Work out the finished part from the listing and answer in its coordinate system (mm). A direction names the side the tool comes from. Round coordinates to 2 decimals unless told otherwise and drop trailing zeros.
1. Flat-ended cylindrical pins translate along their axes: pin 1 Ø0.5 at (x, z) = (0, -3) entering from +Y; pin 2 Ø1.8 at (x, z) = (-2, -2) entering from +Y; pin 3 Ø4 at (x, y) = (2.5, 11.5) entering from -Z. Find the tip coordinate at first contact, or state that the pin passes through.
2. Straight lines are drawn through the part: probe 1 along X at (y, z) = (12, 2); probe 2 along X at (y, z) = (57.5, -2.25); probe 3 along Z at (x, y) = (-0.5, 27.5). For each, find the intervals that lie inside material, in ascending order.
3. A tool of negligible diameter and unlimited length cuts with its end or side. For faces 1 (the face through (-3, 0, 2)), 2 (the face through (-3, 60, 2)), 3 (the face through (3, 0, 2)), 4 (the face through (3, 60, -2)), from which of +Z, -Z, +X, -X, +Y, -Y can it reach the whole face along a straight path? Write none if from no direction.
```python
from build123d import *
from build123d.topology import SkipClean

# Parameters (mm, degrees)
BOSS_EXTRUDE1_DEPTH = 60
SKETCH4_R           = 2.375
BOSS_EXTRUDE3_DEPTH = 2
FILLET1_R           = 0.5
BOSS_EXTRUDE5_START = 2
SKETCH6_R           = 2.375
BOSS_EXTRUDE5_DEPTH = 2
FILLET2_R           = 1


with BuildPart() as part:
    # Sketch2 → Boss-Extrude1 (new body)
    with BuildSketch(Plane(origin=(0, 0, 0), x_dir=(1, 0, 0), z_dir=(0, 1, 0))):
        with BuildLine():
            Line((3.775215965, -0.978645895), (2.300774305, -0.58912019))
            ThreePointArc((2.300774305, -0.58912019), (2.374963211, 0.013219106), (2.294073837, 0.614695232))
            Line((2.294073837, 0.614695232), (3.742962577, 1.0029238))
            ThreePointArc((3.742962577, 1.0029238), (3.356294138, 1.936727823), (2.741299364, 2.73877761))
            Line((2.741299364, 2.73877761), (1.680151223, 1.678605632))
            ThreePointArc((1.680151223, 1.678605632), (1.187973207, 2.056537055), (0.614695232, 2.294073837))
            Line((0.614695232, 2.294073837), (1.0029238, 3.742962577))
            ThreePointArc((1.0029238, 3.742962577), (0, 3.875), (-1.0029238, 3.742962577))
            Line((-1.0029238, 3.742962577), (-0.614695232, 2.294073837))
            ThreePointArc((-0.614695232, 2.294073837), (-1.1875, 2.056810334), (-1.679378605, 1.679378605))
            Line((-1.679378605, 1.679378605), (-2.740038777, 2.740038777))
            ThreePointArc((-2.740038777, 2.740038777), (-3.35584844, 1.9375), (-3.742962577, 1.0029238))
            Line((-3.742962577, 1.0029238), (-2.294073837, 0.614695232))
            ThreePointArc((-2.294073837, 0.614695232), (-2.375, 0), (-2.294073837, -0.614695232))
            Line((-2.294073837, -0.614695232), (-3.742962577, -1.0029238))
            ThreePointArc((-3.742962577, -1.0029238), (-3.35584844, -1.9375), (-2.740038777, -2.740038777))
            Line((-2.740038777, -2.740038777), (-1.679378605, -1.679378605))
            ThreePointArc((-1.679378605, -1.679378605), (-1.1875, -2.056810334), (-0.614695232, -2.294073837))
            Line((-0.614695232, -2.294073837), (-1.0029238, -3.742962577))
            ThreePointArc((-1.0029238, -3.742962577), (0.033967076, -3.874851125), (1.068386506, -3.724805401))
            Line((1.068386506, -3.724805401), (0.681359786, -2.275164575))
            ThreePointArc((0.681359786, -2.275164575), (1.238849907, -2.026296106), (1.714477211, -1.643530618))
            Line((1.714477211, -1.643530618), (2.767163136, -2.698133353))
            ThreePointArc((2.767163136, -2.698133353), (3.500652231, -1.972912562), (3.775215965, -0.978645895))
        make_face()
        Polygon((0.085836926, -0.044584082), (0, 0), (0.073933818, 0), (0.104207494, -0.030328801), (0.080162685, -0.023330742), align=None, mode=Mode.SUBTRACT)
    extrude(amount=BOSS_EXTRUDE1_DEPTH)

    # Sketch4 → Boss-Extrude3 (add)
    with BuildSketch(Plane(origin=(0, 60, 0), x_dir=(1, 0, 0), z_dir=(0, 1, 0))):
        with Locations(Location((0, 0, 0), (0, 0, 75))):
            Circle(SKETCH4_R)
    extrude(amount=BOSS_EXTRUDE3_DEPTH)

    # Fillet1
    # the kernel refuses this fillet: 0.5 mm, written as the material it adds along each edge
    with BuildSketch(Plane(origin=(-2.294073837, 0, 0.614695232), x_dir=(-0.1735157400494046, 0, -0.9848310961556339), z_dir=(0, 1, 0)), Plane(origin=(-1.679378605, 0, -1.679378605), x_dir=(0.7661308776829403, 0, -0.6426845869170722), z_dir=(0, 1, 0)), Plane(origin=(0.614695232, 0, -2.294073837), x_dir=(0.939646617732385, 0, 0.3421465092384974), z_dir=(0, 1, 0)), Plane(origin=(2.294073837, 0, -0.614695232), x_dir=(0.1735157400495284, 0, 0.9848310961556122), z_dir=(0, 1, 0)), Plane(origin=(-0.614695232, 0, 2.294073837), x_dir=(-0.9396466177323688, 0, -0.3421465092385419), z_dir=(0, 1, 0))) as fillet1_piece_1:
        with BuildLine():
            CenterArc((0.458270974, 0.498091484), FILLET1_R, 185.007705084, 79.984589832)
            Line((-0.03982051, 0.45444663), (0, 0))
            ThreePointArc((0, 0), (0.20731306, 0.00906545), (0.414626119, 0))
        make_face()
    extrude(amount=60)
    with BuildSketch(Plane(origin=(-2.294073837, 0, -0.614695232), x_dir=(-0.17351574004940104, 0, 0.9848310961556345), z_dir=(0, 1, 0)), Plane(origin=(-0.614695232, 0, -2.294073837), x_dir=(-0.9396466177323672, 0, 0.3421465092385461), z_dir=(0, 1, 0)), Plane(origin=(1.680151223, 0, -1.678605632), x_dir=(-0.7658350540129166, 0, -0.643037067395833), z_dir=(0, 1, 0))) as fillet1_piece_2:
        with BuildLine():
            CenterArc((0.458270974, -0.498091484), FILLET1_R, 95.007705084, 79.984589832)
            Line((-0.03982051, -0.45444663), (0, 0))
            ThreePointArc((0, 0), (0.20731306, -0.00906545), (0.414626119, 0))
        make_face()
    extrude(amount=60)
    with BuildSketch(Plane(origin=(2.300774305, 0, 0.58912019), x_dir=(0.9668296370387235, 0, 0.2554221073900419), z_dir=(0, 1, 0))) as fillet1_piece_3:
        with BuildLine():
            CenterArc((0.453002414, 0.5), FILLET1_R, 190.38170854, 79.61829146)
            ThreePointArc((-0.038812111, 0.409897433), (-0.010506812, 0.205791362), (0, 0))
            Line((0, 0), (0.453002414, 0))
        make_face()
    extrude(amount=60)
    with BuildSketch(Plane(origin=(1.714477211, 0, 1.643530618), x_dir=(0.7064632978713469, 0, 0.7077496794494086), z_dir=(0, 1, 0))) as fillet1_piece_4:
        with BuildLine():
            CenterArc((0.465508471, -0.5), FILLET1_R, 90, 81.041880237)
            ThreePointArc((-0.02839274, -0.422143763), (-0.00477723, -0.211705398), (0, 0))
            Line((0, 0), (0.465508471, 0))
        make_face()
    extrude(amount=60)
    with BuildSketch(Plane(origin=(0.681359786, 0, 2.275164575), x_dir=(0.25794627414893684, 0, 0.966159262053975), z_dir=(0, 1, 0))) as fillet1_piece_5:
        with BuildLine():
            CenterArc((0.443713653, 0.5), FILLET1_R, 191.464392376, 78.535607624)
            ThreePointArc((-0.046310555, 0.400620549), (-0.014636445, 0.201295026), (0, 0))
            Line((0, 0), (0.443713653, 0))
        make_face()
    extrude(amount=60)
    with BuildSketch(Plane(origin=(-1.679378605, 0, 1.679378605), x_dir=(-0.7071067811865471, 0, 0.707106781186548), z_dir=(0, 1, 0))) as fillet1_piece_6:
        with BuildLine():
            CenterArc((0.456187913, 0.5), FILLET1_R, 190.015410168, 79.984589832)
            ThreePointArc((-0.036192593, 0.413043478), (-0.00906545, 0.20731306), (0, 0))
            Line((0, 0), (0.456187913, 0))
        make_face()
    extrude(amount=60)
    # the kernel refuses this fillet: 0.5 mm, written as the material it takes off along each edge
    with BuildSketch(Plane(origin=(-2.740038777, -1.439160897, 2.740038777), x_dir=(-0.6526300069150477, 0, -0.7576767609436524), z_dir=(0, 1, 0)), Plane(origin=(-3.742962577, -1.439160897, -1.0029238), x_dir=(0.3298523193767966, 0, -0.9440325457322686), z_dir=(0, 1, 0)), Plane(origin=(2.741299364, -1.439160897, -2.73877761), x_dir=(0.652281279601926, 0, 0.7579769998363237), z_dir=(0, 1, 0))) as fillet1_2_piece_1:
        with BuildLine():
            CenterArc((0.538524723, -0.49861874), FILLET1_R, 85.740187873, 98.519624254)
            Line((0.039905983, -0.535758376), (0, 0))
            ThreePointArc((0, 0), (0.287832179, 0.010704768), (0.575664359, 0))
        make_face()
    extrude(amount=62.878321794, mode=Mode.SUBTRACT)
    with BuildSketch(Plane(origin=(-3.742962577, -1.439160897, 1.0029238), x_dir=(0.9659258262890679, 0, -0.2588190451025218), z_dir=(0, 1, 0)), Plane(origin=(-2.740038777, -1.439160897, -2.740038777), x_dir=(0.7071067811865476, 0, 0.7071067811865476), z_dir=(0, 1, 0)), Plane(origin=(3.742962577, -1.439160897, -1.0029238), x_dir=(-0.9659258262890681, 0, 0.25881904510252185), z_dir=(0, 1, 0)), Plane(origin=(-1.0029238, -1.439160897, 3.742962577), x_dir=(0.2588190451025216, 0, -0.9659258262890681), z_dir=(0, 1, 0))) as fillet1_2_piece_2:
        with BuildLine():
            CenterArc((0.537242519, -0.5), FILLET1_R, 90, 98.519624254)
            ThreePointArc((0.04275993, -0.574074074), (0.010704768, -0.287832179), (0, 0))
            Line((0, 0), (0.537242519, 0))
        make_face()
    extrude(amount=62.878321794, mode=Mode.SUBTRACT)
    with BuildSketch(Plane(origin=(-1.0029238, -1.439160897, -3.742962577), x_dir=(0.25881904510252174, 0, 0.965925826289068), z_dir=(0, 1, 0))) as fillet1_2_piece_3:
        with BuildLine():
            CenterArc((0.537242519, 0.5), FILLET1_R, 171.480375746, 98.519624254)
            ThreePointArc((0.04275993, 0.574074074), (0.010704768, 0.287832179), (0, 0))
            Line((0, 0), (0.537242519, 0))
        make_face()
    extrude(amount=62.878321794, mode=Mode.SUBTRACT)
    with BuildSketch(Plane(origin=(1.0029238, -1.439160897, -3.742962577), x_dir=(-0.9824823262918377, 0, -0.1863557847886099), z_dir=(0, 1, 0))) as fillet1_2_piece_4:
        with BuildLine():
            CenterArc((0.538524723, 0.49861874), FILLET1_R, 175.740187873, 98.519624254)
            Line((0.039905983, 0.535758376), (0, 0))
            ThreePointArc((0, 0), (0.287832179, -0.010704768), (0.575664359, 0))
        make_face()
    extrude(amount=62.878321794, mode=Mode.SUBTRACT)
    with BuildSketch(Plane(origin=(3.775215965, -1.264396568, 0.978645895), x_dir=(-0.9668296370387236, 0, -0.25542210739004173), z_dir=(0, 1, 0))) as fillet1_2_piece_5:
        with BuildLine():
            CenterArc((0.437999819, 0.5), FILLET1_R, 179.77718135, 90.22281865)
            ThreePointArc((-0.0619964, 0.501944455), (-0.046928547, 0.249004631), (0, 0))
            Line((0, 0), (0.437999819, 0))
        make_face()
    extrude(amount=62.528793137, mode=Mode.SUBTRACT)
    with BuildSketch(Plane(origin=(2.767163136, -1.241563867, 2.698133353), x_dir=(0.8000663385432955, 0, -0.5999115384203949), z_dir=(0, 1, 0))) as fillet1_2_piece_6:
        with BuildLine():
            CenterArc((0.434547354, 0.496131331), FILLET1_R, 188.084320914, 89.047719887)
            Line((-0.060483736, 0.425816179), (0, 0))
            ThreePointArc((0, 0), (0.248312773, -0.015474675), (0.496625547, 0))
        make_face()
    extrude(amount=62.483127735, mode=Mode.SUBTRACT)
    with BuildSketch(Plane(origin=(1.068386506, -1.410819518, 3.724805401), x_dir=(-0.9787647804449897, 0, 0.20498659605074468), z_dir=(0, 1, 0))) as fillet1_2_piece_7:
        with BuildLine():
            CenterArc((0.527919562, -0.498672678), FILLET1_R, 85.824226653, 97.295295094)
            Line((0.028660468, -0.525882193), (0, 0))
            ThreePointArc((0, 0), (0.282163904, 0.010286747), (0.564327807, 0))
        make_face()
    extrude(amount=62.821639036, mode=Mode.SUBTRACT)

    # Sketch6 → Boss-Extrude5 (add)
    with SkipClean():  # the faces are left unmerged after this step: merging them gives an invalid solid
        with BuildSketch(Plane.XZ.offset(BOSS_EXTRUDE5_START)):
            with Locations(Location((0, 0, 0), (0, 0, 270))):
                Circle(SKETCH6_R)
        extrude(amount=-BOSS_EXTRUDE5_DEPTH)

    # Fillet2
    fillet2_edges = [part.edges().sort_by_distance(p)[0] for p in [
        (-0.614695232, 62, 2.294073837),
        (0, -2, 2.375),
    ]]
    fillet(fillet2_edges, radius=FILLET2_R)


solid = part.part
```
Worked answers:
1. pin 1: stops at y = 60
1. pin 2: stops at y = 61.83
1. pin 3: stops at z = -3.84
2. probe 1: x = -3.32 to -2, -1.28 to 1.28, 2.07 to 3.48
2. probe 2: x = -3.15 to -2.25, -0.86 to 0.86, 2.25 to 3.15
2. probe 3: z = -3.84 to 3.84
3. face 1: +Z, -X, -Y
3. face 2: +Z, -X, +Y
3. face 3: +Z, +X, -Y
3. face 4: -Z, +X, +Y
